Verification items for the finished model (mm, model axes). A direction names the side the tool comes from. Round coordinates to 2 decimals unless told otherwise and drop trailing zeros. Write each loop counter-clockwise with the first axis right and the second up, starting at its lowest first coordinate (ties: lowest second). Pieces come first, ordered by that corner, then holes. Notation, with made-up numbers: M -18.5,-0.75 L 4.5,-0.75 A21 cw 4.5,30.25 Z; hole C 70,1.25 d8. An arc over 180 degrees is marked long. One line per question, with ' | ' between items.
from build123d import *

# Parameters (mm, degrees)
CROQUIS1_W              = 160
CROQUIS1_H              = 45.5
SALIENTE_EXTRUIR1_DEPTH = 25
CROQUIS2_W              = 160
CROQUIS2_H              = 45.5
SALIENTE_EXTRUIR2_DEPTH = 2
CROQUIS5_R              = 13
CORTAR_EXTRUIR3_DEPTH   = 2
CORTAR_EXTRUIR4_REACH   = 8
CROQUIS6_W              = 20
CROQUIS6_H              = 25
REDONDEO1_R             = 5
REDONDEO2_R             = 5
CORTAR_EXTRUIR5_REACH   = 8
CROQUIS7_R              = 2.3
CORTAR_EXTRUIR6_REACH   = 8
CROQUIS8_R              = 2.3
CORTAR_EXTRUIR7_REACH   = 47.5
CROQUIS9_R              = 2.3
CROQUIS10_R             = 2.3
CORTAR_EXTRUIR8_DEPTH   = 20
CROQUIS11_R             = 2.3
CORTAR_EXTRUIR9_DEPTH   = 20


with BuildPart() as part:
    # Croquis1 → Saliente-Extruir1 (new body)
    with BuildSketch(Plane.XY):
        Rectangle(CROQUIS1_W, CROQUIS1_H)
        Polygon((-33.600403232, 16.75), (33.600403232, 16.75), (46, 10.25), (41.5, -16.75), (-41.5, -16.75), (-46, 10.25), align=None, mode=Mode.SUBTRACT)
    extrude(amount=SALIENTE_EXTRUIR1_DEPTH)

    # Croquis2 → Saliente-Extruir2 (add)
    with BuildSketch(Plane(origin=(0, 0, 0), x_dir=(-1, 0, 0), z_dir=(0, 0, -1))):
        Rectangle(CROQUIS2_W, CROQUIS2_H)
    extrude(amount=SALIENTE_EXTRUIR2_DEPTH)

    # Croquis5 → Cortar-Extruir3 (cut)
    with BuildSketch(Plane.XY):
        with Locations((0, 1.75)):
            Circle(CROQUIS5_R)
    extrude(amount=-CORTAR_EXTRUIR3_DEPTH, mode=Mode.SUBTRACT)

    # Croquis6 → Cortar-Extruir4 (cut, up to next)
    with BuildSketch(Plane(origin=(0, -16.75, 0), x_dir=(1, 0, 0), z_dir=(0, 1, 0)), mode=Mode.PRIVATE) as cortar_extruir4_sk1:
        with Locations((0, -12.5)):
            Rectangle(CROQUIS6_W, CROQUIS6_H)
    cortar_extruir4_tool1 = extrude(cortar_extruir4_sk1.sketch, amount=-CORTAR_EXTRUIR4_REACH, mode=Mode.PRIVATE) & part.part
    add(cortar_extruir4_tool1.solids().sort_by_distance((0, -16.75, 12.5))[0], mode=Mode.SUBTRACT)

    # Redondeo1
    redondeo1_edges = [part.edges().sort_by_distance(p)[0] for p in [
        (-10, -19.75, 0),
        (10, -19.75, 0),
    ]]
    fillet(redondeo1_edges, radius=REDONDEO1_R)

    # Redondeo2
    redondeo2_edges = [part.edges().sort_by_distance(p)[0] for p in [
        (-10, -19.75, 25),
        (10, -19.75, 25),
    ]]
    fillet(redondeo2_edges, radius=REDONDEO2_R)

    # Croquis7 → Cortar-Extruir5 (cut, up to next)
    with BuildSketch(Plane(origin=(0, -16.75, 0), x_dir=(1, 0, 0), z_dir=(0, 1, 0)), mode=Mode.PRIVATE) as cortar_extruir5_sk1:
        with Locations((-31.5, -8)):
            Circle(CROQUIS7_R)
    cortar_extruir5_tool1 = extrude(cortar_extruir5_sk1.sketch, amount=-CORTAR_EXTRUIR5_REACH, mode=Mode.PRIVATE) & part.part
    add(cortar_extruir5_tool1.solids().sort_by_distance((-31.5, -16.75, 8))[0], mode=Mode.SUBTRACT)
    # Croquis7 → Cortar-Extruir5 (cut, up to next)
    with BuildSketch(Plane(origin=(0, -16.75, 0), x_dir=(1, 0, 0), z_dir=(0, 1, 0)), mode=Mode.PRIVATE) as cortar_extruir5_sk2:
        with Locations((31.5, -8)):
            Circle(CROQUIS7_R)
    cortar_extruir5_tool2 = extrude(cortar_extruir5_sk2.sketch, amount=-CORTAR_EXTRUIR5_REACH, mode=Mode.PRIVATE) & part.part
    add(cortar_extruir5_tool2.solids().sort_by_distance((31.5, -16.75, 8))[0], mode=Mode.SUBTRACT)

    # Croquis8 → Cortar-Extruir6 (cut, up to next)
    with BuildSketch(Plane.XZ.offset(-16.75), mode=Mode.PRIVATE) as cortar_extruir6_sk1:
        with Locations((-28.600403232, 8)):
            Circle(CROQUIS8_R)
    cortar_extruir6_tool1 = extrude(cortar_extruir6_sk1.sketch, amount=-CORTAR_EXTRUIR6_REACH, mode=Mode.PRIVATE) & part.part
    add(cortar_extruir6_tool1.solids().sort_by_distance((-28.600403, 16.75, 8))[0], mode=Mode.SUBTRACT)
    # Croquis8 → Cortar-Extruir6 (cut, up to next)
    with BuildSketch(Plane.XZ.offset(-16.75), mode=Mode.PRIVATE) as cortar_extruir6_sk2:
        with Locations((28.600403232, 8)):
            Circle(CROQUIS8_R)
    cortar_extruir6_tool2 = extrude(cortar_extruir6_sk2.sketch, amount=-CORTAR_EXTRUIR6_REACH, mode=Mode.PRIVATE) & part.part
    add(cortar_extruir6_tool2.solids().sort_by_distance((28.600403, 16.75, 8))[0], mode=Mode.SUBTRACT)

    # Croquis9 → Cortar-Extruir7 (cut, up to next)
    with BuildSketch(Plane(origin=(0, 22.75, 0), x_dir=(1, 0, 0), z_dir=(0, 1, 0)), mode=Mode.PRIVATE) as cortar_extruir7_sk1:
        with Locations((-10, -4)):
            Circle(CROQUIS9_R)
    cortar_extruir7_tool1 = extrude(cortar_extruir7_sk1.sketch, amount=-CORTAR_EXTRUIR7_REACH, mode=Mode.PRIVATE) & part.part
    add(cortar_extruir7_tool1.solids().sort_by_distance((-10, 22.75, 4))[0], mode=Mode.SUBTRACT)
    # Croquis9 → Cortar-Extruir7 (cut, up to next)
    with BuildSketch(Plane(origin=(0, 22.75, 0), x_dir=(1, 0, 0), z_dir=(0, 1, 0)), mode=Mode.PRIVATE) as cortar_extruir7_sk2:
        with Locations((10, -4)):
            Circle(CROQUIS9_R)
    cortar_extruir7_tool2 = extrude(cortar_extruir7_sk2.sketch, amount=-CORTAR_EXTRUIR7_REACH, mode=Mode.PRIVATE) & part.part
    add(cortar_extruir7_tool2.solids().sort_by_distance((10, 22.75, 4))[0], mode=Mode.SUBTRACT)
    # Croquis9 → Cortar-Extruir7 (cut, up to next)
    with BuildSketch(Plane(origin=(0, 22.75, 0), x_dir=(1, 0, 0), z_dir=(0, 1, 0)), mode=Mode.PRIVATE) as cortar_extruir7_sk3:
        with Locations((0, -17)):
            Circle(CROQUIS9_R)
    cortar_extruir7_tool3 = extrude(cortar_extruir7_sk3.sketch, amount=-CORTAR_EXTRUIR7_REACH, mode=Mode.PRIVATE) & part.part
    add(cortar_extruir7_tool3.solids().sort_by_distance((0, 22.75, 17))[0], mode=Mode.SUBTRACT)

    # Croquis10 → Cortar-Extruir8 (cut)
    with BuildSketch(Plane.ZY.offset(80)):
        with Locations((11.5, 0)):
            Circle(CROQUIS10_R)
        with Locations((11.5, -12.75)):
            Circle(CROQUIS10_R)
        with Locations((11.5, 12.75)):
            Circle(CROQUIS10_R)
    extrude(amount=-CORTAR_EXTRUIR8_DEPTH, mode=Mode.SUBTRACT)

    # Croquis11 → Cortar-Extruir9 (cut)
    with BuildSketch(Plane(origin=(80, 0, 0), x_dir=(0, 0, -1), z_dir=(1, 0, 0))):
        with Locations((-11.5, 12.75)):
            Circle(CROQUIS11_R)
        with Locations((-11.5, 0)):
            Circle(CROQUIS11_R)
        with Locations((-11.5, -12.75)):
            Circle(CROQUIS11_R)
    extrude(amount=-CORTAR_EXTRUIR9_DEPTH, mode=Mode.SUBTRACT)


solid = part.part
1. Thickness scan on line 1 (Y direction, x = -75, z = 11.5); line 2 (X direction, y = -21.3, z = 8); line 3 (X direction, y = 18.8, z = 4). Record the ranges inside material, lowest first.
Results:
line 1: y = -22.75 to -15.05, -10.45 to -2.3, 2.3 to 10.45, 15.05 to 22.75 | line 2: x = -80 to -33.8, -29.2 to -10, 10 to 29.2, 33.8 to 80 | line 3: x = -80 to -12.3, -7.7 to 7.7, 12.3 to 80
2. Tool access check on faces 1 (the face through (60, -13, 12)), 2 (the face through (-9, -20, 2)), 3 (the face through (29.837, 19.708, 9.939)). Record the directions out of +Z, -Z, +X, -X, +Y, -Y that give a thin tool (end or side, any length) a straight path to the whole face; none if there is none.
Results:
face 1: +X | face 2: +Z, -Y | face 3: +Y
3. Section check D-D, the plane y = 12.75. Record the cut outline in (x, z).
Results:
outline: M -80,-2 L -6.93,-2 L -6.93,0 L -41.23,0 L -41.23,25 L -80,25 L -80,13.8 L -60,13.8 L -60,9.2 L -80,9.2 Z; M 6.93,-2 L 80,-2 L 80,9.2 L 60,9.2 L 60,13.8 L 80,13.8 L 80,25 L 41.23,25 L 41.23,0 L 6.93,0 Z
4. Section check B-B, the plane x = 23. Record the cut outline in (y, z), then the cut area to 3 significant figures.
Results:
outline: M -22.75,-2 L 22.75,-2 L 22.75,25 L 16.75,25 L 16.75,0 L -16.75,0 L -16.75,25 L -22.75,25 Z | area: 391 mm2
5. Section check C-C, the plane y = -4.5. Record the cut outline in (x, z).
Results:
outline: M -80,-2 L -11.4,-2 L -11.4,0 L -43.54,0 L -43.54,25 L -80,25 Z; M 11.4,-2 L 80,-2 L 80,25 L 43.54,25 L 43.54,0 L 11.4,0 Z
6. Mould release check, pull along Y, two halves, no side actions. Record for faces 4 (the face through (-10.316, -6.16, -0.986)), 5 (the face through (-1, 21, 25)): pulls with the +Y half, pulls with the -Y half, needs draft (parallel to the pull), parting line crosses it, or undercut.
Results:
face 4: undercut | face 5: needs draft
7. Go/stop test with flat-tipped pins: P1, Ø3.5, axis at x = 31.5, z = 8, coming from the -Y side; P2, Ø3.5, axis at y = 0, z = 11.5, coming from the +X side. Record where each tip stops, or that it passes through.
Results:
P1: stops at y = 16.75 | P2: stops at x = 60
8. Section check A-A, the plane y = 4.5. Record the cut outline in (x, z), then the cut area to 3 significant figures.
Results:
outline: M -80,-2 L -12.71,-2 L -12.71,0 L -45.04,0 L -45.04,25 L -80,25 Z; M 12.71,-2 L 80,-2 L 80,25 L 45.04,25 L 45.04,0 L 12.71,0 Z | area: 2,020 mm2
